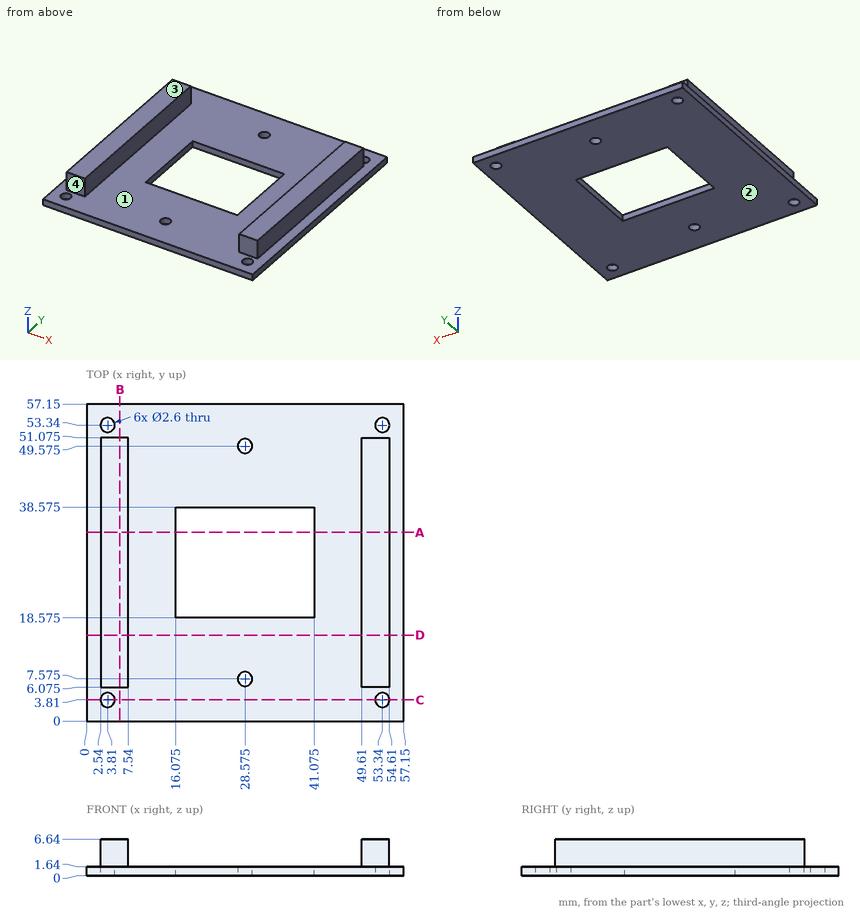
Could you check a few things on this drawing? It's one solid part, dimensions in mm from its lowest x, y, z. A direction names the side the tool comes from. Round coordinates to 2 decimals unless told otherwise and drop trailing zeros. Write each loop counter-clockwise with the first axis right and the second up, starting at its lowest first coordinate (ties: lowest second). Pieces come first, ordered by that corner, then holes. Notation, with made-up numbers: M 87.5,49.25 L 98.5,49.25 A18 cw 98.5,58.25 Z; hole C 1,-36.5 d3. An arc over 180 degrees is marked long. Answer as CSV lines item,"result". Start each with the question number.
1. Suppose I cut it at C-C on y = 3.81. Write out the boundary of the cut face in (x, z).
2. Suppose I cut it at B-B on x = 6. Write out the boundary of the cut face in (y, z) (3 decimals), then the cut area to 3 significant figures.
3. I need wall thicknesses on probe 1 along Y at (x, z) = (3.81, 1.3); probe 2 along X at (y, z) = (20, 1.5) (3 decimals); probe 3 along X at (y, z) = (4.5, 1). Which ranges of each line are inside material? Lowest first, please.
4. Suppose I cut it at D-D on y = 15.5. Write out the boundary of the cut face in (x, z).
5. Thinking about a two-plate mould opening in X: for the marked faces 1 and 2, which applies, released by +X, released by -X, zero draft, split by the parting line, or undercut?
6. Suppose I cut it at A-A on y = 34. Write out the boundary of the cut face in (x, z) (3 decimals).
7. I'm going to push flat-ended pins straight in: pin 1 Ø2.5 at (x, y) = (3.81, 53.34) entering from -Z; pin 2 Ø2.5 at (y, z) = (31, 4) entering from +X; pin 3 Ø10 at (x, y) = (38.5, 31.5) entering from +Z; pin 4 Ø3 at (y, z) = (20, 3) entering from +X. Where does each tip first touch, or does it pass through?
8. On a 3-axis mill with a long thin cutter (end or side, diameter ignored), from which of +Z, -Z, +X, -X, +Y, -Y can I reach the whole of each face in a straight line? I mean the marked faces 3 and 4. Say none if no direction works.
Check result:
1,outline,"M 0,0 L 2.51,0 L 2.51,1.64 L 0,1.64 Z; M 5.11,0 L 52.04,0 L 52.04,1.64 L 5.11,1.64 Z; M 54.64,0 L 57.15,0 L 57.15,1.64 L 54.64,1.64 Z"
2,outline,"M 0,0 L 57.15,0 L 57.15,1.64 L 51.075,1.64 L 51.075,6.64 L 6.075,6.64 L 6.075,1.64 L 0,1.64 Z"
2,area,"319 mm2"
3,probe 1,"y = 0 to 2.51, 5.11 to 52.04, 54.64 to 57.15"
3,probe 2,"x = 0 to 16.075, 41.075 to 57.15"
3,probe 3,"x = 0 to 2.71, 4.91 to 52.24, 54.44 to 57.15"
4,outline,"M 0,0 L 57.15,0 L 57.15,1.64 L 54.61,1.64 L 54.61,6.64 L 49.61,6.64 L 49.61,1.64 L 7.54,1.64 L 7.54,6.64 L 2.54,6.64 L 2.54,1.64 L 0,1.64 Z"
5,face 1,"undercut"
5,face 2,"zero draft"
6,outline,"M 0,0 L 16.075,0 L 16.075,1.64 L 7.54,1.64 L 7.54,6.64 L 2.54,6.64 L 2.54,1.64 L 0,1.64 Z; M 41.075,0 L 57.15,0 L 57.15,1.64 L 54.61,1.64 L 54.61,6.64 L 49.61,6.64 L 49.61,1.64 L 41.075,1.64 Z"
7,pin 1,"passes through"
7,pin 2,"stops at x = 54.61"
7,pin 3,"stops at z = 1.64"
7,pin 4,"stops at x = 57.15"
8,face 3,"+Z, +X, -X, +Y, -Y"
8,face 4,"+Z, +X, -X, -Y"
